Part model, mm, in its own coordinate system. Round coordinates to 2 decimals unless told otherwise and drop trailing zeros. Loops run counter-clockwise (first coordinate to the right, second up) from the corner with the lowest first, then second, coordinate; pieces in that order, holes last. Notation, with made-up numbers: M 60.5,-33 L 84.5,-33 A25 ccw 84.5,-21 Z; hole C -6,72 d1. An arc over 180 degrees is marked long. Put each result on its own line as item: value. Start each with the question number.
```python
from build123d import *

# Parameters (mm, degrees)
SKETCH1_R           = 6.75
SKETCH1_R_2         = 1.25
BOSS_EXTRUDE1_DEPTH = 1.75


with BuildPart() as part:
    # Sketch1 → Boss-Extrude1 (new body, symmetric)
    with BuildSketch(Plane.XY):
        Circle(SKETCH1_R)
        Circle(SKETCH1_R_2, mode=Mode.SUBTRACT)
    extrude(amount=BOSS_EXTRUDE1_DEPTH, both=True)

    # Sketch2 one side → Cut-Revolve1 (revolve, cut)
    with BuildSketch(Plane(origin=(0, 0, 0), x_dir=(1, 0, 0), z_dir=(0, 1, 0))):
        with BuildLine():
            Line((6.75, 1.75), (0, 1.75))
            Line((0, 1.75), (0, 0.772873706))
            ThreePointArc((0, 0.772873706), (3.410178727, 1.018421792), (6.75, 1.75))
        make_face()
    cut_revolve1 = revolve(axis=Axis((0, 0, -3.982137232), (0, 0, 1)), mode=Mode.SUBTRACT)

    # Mirror1: Cut-Revolve1 across plane
    add(cut_revolve1.mirror(Plane.XY), mode=Mode.SUBTRACT)


solid = part.part
```
1. Cut at A-A, the plane y = 0. Give the cut face in (x, z).
2. Cut at C-C, the plane z = -0.15. Give the cut face in (x, y).
3. Drop flat-ended pins along their axis: pin 1 (1.5 mm diameter, centred on x = 1, z = -0.5, fed in from -Y); pin 2 (5 mm diameter, centred on x = -1, y = -3, fed in from -Z); pin 3 (4 mm diameter, centred on x = 0, y = 0, fed in from -Z); pin 4 (2 mm diameter, centred on y = 0.5, z = 1, fed in from -X). Give the stop position or say it passes through.
4. Cut at D-D, the plane x = 4.75. Give the cut face in (y, z).
5. Mould opens along X. For faces 1 (the cylindrical face through (-1.46, -6.59, 0.02)), 2 (the cylindrical face through (-0.27, -1.22, -0.01)) say: released by +X, released by -X, zero draft, split by the parting line, or undercut.
6. Wall check: L1, parallel to Y at x = 0, z = -0.1; L2, parallel to Y at x = -1, z = -0.75; L3, parallel to X at y = -6, z = -0.35. Give the ranges that are in metal, low to high.
Results list:
1. outline: M -6.75,-1.75 A23.8 cw -1.25,-0.81 L -1.25,0.81 A23.8 cw -6.75,1.75 Z; M 1.25,-0.81 A23.8 cw 6.75,-1.75 L 6.75,1.75 A23.8 cw 1.25,0.81 Z
2. outline: C 0,0 d13.5; hole C 0,0 d2.5
3. pin 1: stops at y = -6.75
3. pin 2: stops at z = -1.46
3. pin 3: stops at z = -0.86
3. pin 4: stops at x = -6.75
4. outline: M -4.8,-1.75 A23.32 cw 4.8,-1.75 L 4.8,1.75 A23.32 cw -4.8,1.75 Z
5. face 1: split by the parting line
5. face 2: undercut
6. L1: y = -6.75 to -1.25, 1.25 to 6.75
6. L2: y = -6.68 to -0.75, 0.75 to 6.68
6. L3: x = -3.09 to 3.09
